Design review of the part built by this model. Coordinates are the model's own, in mm. Give positions to 0.01 mm unless a question says otherwise; leave off trailing zeros. Loops run counter-clockwise (first coordinate to the right, second up) from the corner with the lowest first, then second, coordinate; pieces in that order, holes last. Notation, with made-up numbers: (-40, 48.5) - (-28, 48.5) arc R31 ccw to (-28, 76.5) - close; hole circle Ø5 at (22, 12). An arc over 180 degrees is marked (long way). Write each question's results on one line, items separated by ' | '.
```python
from build123d import *

# Parameters (mm, degrees)
SKETCH1_R          = 8
SKETCH1_R_2        = 5
SKETCH1_R_3        = 2.25
SKETCH1_R_4        = 3
EXTRUDE1_DEPTH     = 20
SKETCH3_R          = 8
CUT_EXTRUDE2_DEPTH = 10
SKETCH4_R          = 3.25
CUT_EXTRUDE3_DEPTH = 60
SKETCH5_R          = 5
CUT_EXTRUDE4_DEPTH = 6


with BuildPart() as part:
    # Sketch1 → Extrude1 (new body)
    with BuildSketch(Plane.XY):
        Polygon((-20, 229.5), (38.999908, 439.49994136), (180, 439.50001453), (180, 30), (180, 0), (-20, 0), (-20, 30), align=None)
        with Locations((126.999908, 339.49994136)):
            Circle(SKETCH1_R, mode=Mode.SUBTRACT)
        with Locations((157.49992067, 416.99997068)):
            Circle(SKETCH1_R_2, mode=Mode.SUBTRACT)
        with Locations((126.999908, 363.49994136)):
            Circle(SKETCH1_R_3, mode=Mode.SUBTRACT)
        with Locations((126.999908, 315.49994136)):
            Circle(SKETCH1_R_3, mode=Mode.SUBTRACT)
        with Locations((157.49992067, 261.99991204)):
            Circle(SKETCH1_R_2, mode=Mode.SUBTRACT)
        with Locations((126.12492067, 261.99991204)):
            Circle(SKETCH1_R_4, mode=Mode.SUBTRACT)
        with Locations((126.12492067, 416.99997068)):
            Circle(SKETCH1_R_4, mode=Mode.SUBTRACT)
    extrude(amount=EXTRUDE1_DEPTH)

    # Sketch3 → Cut-Extrude2 (cut)
    with BuildSketch(Plane.XY.offset(20)):
        with Locations((157.49992067, 416.99997068)):
            Circle(SKETCH3_R)
        with Locations((157.49992067, 261.99991204)):
            Circle(SKETCH3_R)
    extrude(amount=-CUT_EXTRUDE2_DEPTH, mode=Mode.SUBTRACT)

    # Sketch4 → Cut-Extrude3 (cut)
    with BuildSketch(Plane.XZ):
        with Locations((20, 10)):
            Circle(SKETCH4_R)
        with Locations((40, 10)):
            Circle(SKETCH4_R)
        with Locations((60, 10)):
            Circle(SKETCH4_R)
        with Locations((80, 10)):
            Circle(SKETCH4_R)
        with Locations((100, 10)):
            Circle(SKETCH4_R)
        with Locations((120, 10)):
            Circle(SKETCH4_R)
        with Locations((140, 10)):
            Circle(SKETCH4_R)
        with Locations((160, 10)):
            Circle(SKETCH4_R)
        with Locations((0, 10)):
            Circle(SKETCH4_R)
    extrude(amount=-CUT_EXTRUDE3_DEPTH, mode=Mode.SUBTRACT)

    # Sketch5 → Cut-Extrude4 (cut)
    with BuildSketch(Plane.XY.offset(20)):
        with Locations((126.12492067, 416.99997068)):
            Circle(SKETCH5_R)
        with Locations((126.12492067, 261.99991204)):
            Circle(SKETCH5_R)
    extrude(amount=-CUT_EXTRUDE4_DEPTH, mode=Mode.SUBTRACT)


solid = part.part
```
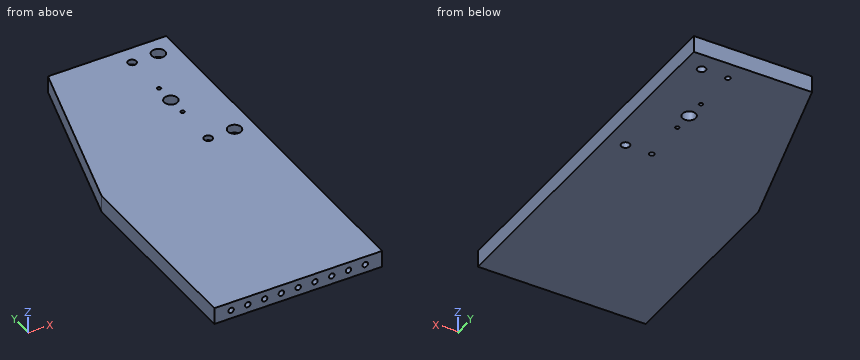
Item 1: Clearance check with flat-ended pins moving along their axes: P1, Ø2, axis at x = 81, z = 11.5, coming from the -Y side; P2, Ø13, axis at x = 157.5, y = 262, coming from the +Z side; P3, Ø7.5, axis at x = 0, z = 10, coming from the -Y side; P4, Ø6, axis at y = 321, z = 16, coming from the -X side. State where each tip first meets the part, or that it passes through.
Output values:
P1: stops at y = 60 | P2: stops at z = 10 | P3: stops at y = 0 | P4: stops at x = 4.86
Item 2: Wall thickness on probe 1 along Z at (x, y) = (40, 33); probe 2 along X at (y, z) = (262, 12.25); probe 3 along X at (y, z) = (348, 12.25): over which ranges is each line inside the solid? List them lowest first.
Output values:
probe 1: z = 0 to 6.75, 13.25 to 20 | probe 2: x = -10.87 to 123.12, 129.12 to 149.5, 165.5 to 180 | probe 3: x = 13.29 to 180
Item 3: We need section A-A on z = 3. Give the boundary of the cut face in (x, y).
Output values:
outline: (-20, 0) - (180, 0) - (180, 439.5) - (39, 439.5) - (-20, 229.5) - close; hole circle Ø16 at (127, 339.5); hole circle Ø6 at (126.12, 262); hole circle Ø6 at (126.12, 417); hole circle Ø4.5 at (127, 315.5); hole circle Ø4.5 at (127, 363.5); hole circle Ø10 at (157.5, 262); hole circle Ø10 at (157.5, 417)
